Input: part model. Units: mm. Frame: model coordinates. A direction names the side the tool comes from. Give positions to 0.01 mm unless a question says otherwise; leave off trailing zeros. Loops run counter-clockwise (first coordinate to the right, second up) from the corner with the lowest first, then second, coordinate; pieces in that order, holes last. Notation, with made-up numbers: M -6.75,-35 L 30.25,-35 A25 ccw 30.25,0 Z; hole C 51,2.5 d6. An arc over 180 degrees is marked long. Answer as a JSON object with one key per item and string values. Group by question number.
1) Access query for faces 1 (the flat face through (2251.712, 700, 381)), 2 (the flat face through (2251.712, 683, 479)), 3 (the cylindrical face through (2298.4, 703.4, 400)), 4 (the flat face through (2280, 687.227, 517)). Directions: +Z, -Z, +X, -X, +Y, -Y. A direction counts if a zero-diameter tool reaches every point of the face in a straight line with its end or side. Return the directions, or none.
2) Section query D-D on z = 455. Return loops of the section in (x, y).
3) Section query B-B on z = 340.5. Return loops of the section in (x, y).
4) First-contact query: P1, Ø16.5, axis at x = 2271, z = 516.5, coming from the +Y side; P2, Ø10, axis at x = 2292.35, y = 701.47, coming from the +Z side; P3, Ø6, axis at y = 678, z = 319, coming from the +X side; P4, Ø19, axis at x = 2301.5, y = 694, coming from the -Z side. Flat tips, straight axial feed; report the tip coordinate or a pass-through.
5) Section query C-C on z = 275.59. Return loops of the section in (x, y).
6) Section query A-A on x = 2257. Return loops of the section in (y, z), plus the area to 3 significant figures.
7) Draft query along X for faces 5 (the cylindrical face through (2298.4, 703.4, 361.3)), 6 (the flat face through (2260.71, 699.83, 312.56)), 7 (the flat face through (2290.21, 671.3, 451.21)), 8 (the flat face through (2292, 686.862, 328)). Return one class per face: +X half, -X half, draft (parallel to the pull), parting line (faces both ways), or undercut.
8) Ray query, L1, parallel to Z at x = 2275, y = 699; L2, parallel to X at y = 698.5, z = 370.5; L3, parallel to Z at x = 2258.5, y = 714. Return the intervals inside material, ascending.
from build123d import *

# Parameters (mm, degrees)
SKETCH1_R                      = 15
SKETCH1_W                      = 81.28
SKETCH1_H                      = 29.9212
BOSS_EXTRUDE1_DEPTH            = 88.9
CUT_EXTRUDE1_DEPTH             = 894.223960082
CUT_EXTRUDE1_DEPTH_BACK        = 894.223960082
CUT_EXTRUDE2_REACH             = 2404.418
CUT_EXTRUDE2_DIRECTION_2_DEPTH = 2403.418387278
CUT_EXTRUDE3_DEPTH             = 2403.418387278
CUT_EXTRUDE3_DEPTH_BACK        = 31.75
SKETCH6_R                      = 6.35
CUT_EXTRUDE4_DEPTH             = 31.75
SKETCH7_R                      = 6.35
CUT_EXTRUDE5_DEPTH             = 50.8


with BuildPart() as part:
    # Sketch1 → Boss-Extrude1 (new body)
    with BuildSketch(Plane(origin=(0, 718.612000035, 0), x_dir=(1, 0, 0), z_dir=(0, 1, 0))):
        with BuildLine():
            Line((2295.073740346, -527.28515435), (2266.117740346, -527.28515435))
            Line((2266.117740346, -527.28515435), (2241.551712769, -484.433115091))
            Line((2241.551712769, -484.433115091), (2241.551712769, -356.772715091))
            Line((2241.551712769, -356.772715091), (2280.410248463, -267.100940225))
            ThreePointArc((2280.410248463, -267.100940225), (2301.649946984, -254.303850194), (2320.663918503, -270.221111063))
            Line((2320.663918503, -270.221111063), (2343.151712769, -356.772715091))
            Line((2343.151712769, -356.772715091), (2343.151712769, -404.372315091))
            Line((2343.151712769, -404.372315091), (2319.639767922, -484.433115091))
            Line((2319.639767922, -484.433115091), (2295.073740346, -527.28515435))
        make_face()
        with Locations(Location((2299.99999994, -275.59, 0), (0, 0, 270))):
            Circle(SKETCH1_R, mode=Mode.SUBTRACT)
        with Locations((2292.351712769, -380.572515091)):
            Rectangle(SKETCH1_W, SKETCH1_H, mode=Mode.SUBTRACT)
    extrude(amount=-BOSS_EXTRUDE1_DEPTH)

    # Sketch3 → Cut-Extrude1 (cut, two sides: drawn at the far end of the back side and taken through both)
    with BuildSketch(Plane(origin=(2299.99999994, 0, 0), x_dir=(0, 0, -1), z_dir=(1, 0, 0)).offset(-CUT_EXTRUDE1_DEPTH_BACK)):
        Polygon((-254.240000028, 680.512000035), (-414.278315091, 680.512000035), (-489.18515435, 661.827103465), (-527.28515435, 661.827103465), (-527.28515435, 629.712000035), (-254.240000028, 629.712000035), align=None)
        Polygon((-527.28515435, 687.227103465), (-527.28515435, 718.612000035), (-400.308315091, 718.612000035), (-506.96515435, 687.227103465), align=None)
    extrude(amount=CUT_EXTRUDE1_DEPTH + CUT_EXTRUDE1_DEPTH_BACK, mode=Mode.SUBTRACT)

    # Cut-Extrude2: up to this plane
    cut_extrude2_end = Plane(origin=(2241.551712769, 686.673213286, 415.815179194), z_dir=(0, 0.9702698033545601, 0.24202584303810049))
    # Sketch4 → Cut-Extrude2 (cut, up to the surface)
    with BuildSketch(Plane(origin=(0, 718.612000035, 0), x_dir=(1, 0, 0), z_dir=(0, 1, 0)), mode=Mode.PRIVATE) as cut_extrude2_sk1:
        Polygon((2317.374261561, -469.611817535), (2336.533545297, -404.372315091), (2251.711712769, -404.372315091), (2251.711712769, -469.611817535), align=None)
    cut_extrude2_tool1 = split(extrude(cut_extrude2_sk1.sketch, amount=-CUT_EXTRUDE2_REACH, mode=Mode.PRIVATE), bisect_by=cut_extrude2_end, keep=Keep.BOTH, mode=Mode.PRIVATE)
    add(cut_extrude2_tool1.solids().sort_by_distance((2289.536084, 718.612, 435.607712))[0], mode=Mode.SUBTRACT)
    # Sketch4 → Cut-Extrude2 (cut, up to the surface)
    with BuildSketch(Plane(origin=(0, 718.612000035, 0), x_dir=(1, 0, 0), z_dir=(0, 1, 0)), mode=Mode.PRIVATE) as cut_extrude2_sk2:
        Polygon((2313.02160045, -484.433115091), (2315.882386888, -474.691817535), (2251.711712769, -474.691817535), (2251.711712769, -484.433115091), (2264.6287806, -506.96515435), (2300.104532619, -506.96515435), align=None)
    cut_extrude2_tool2 = split(extrude(cut_extrude2_sk2.sketch, amount=-CUT_EXTRUDE2_REACH, mode=Mode.PRIVATE), bisect_by=cut_extrude2_end, keep=Keep.BOTH, mode=Mode.PRIVATE)
    add(cut_extrude2_tool2.solids().sort_by_distance((2282.625495, 718.612, 489.24748))[0], mode=Mode.SUBTRACT)

    # Sketch4 → Cut-Extrude2 direction 2 (cut)
    with BuildSketch(Plane(origin=(0, 718.612000035, 0), x_dir=(1, 0, 0), z_dir=(0, 1, 0))):
        Polygon((2317.374261561, -469.611817535), (2336.533545297, -404.372315091), (2251.711712769, -404.372315091), (2251.711712769, -469.611817535), align=None)
        Polygon((2313.02160045, -484.433115091), (2315.882386888, -474.691817535), (2251.711712769, -474.691817535), (2251.711712769, -484.433115091), (2264.6287806, -506.96515435), (2300.104532619, -506.96515435), align=None)
    extrude(amount=CUT_EXTRUDE2_DIRECTION_2_DEPTH, mode=Mode.SUBTRACT)

    # Sketch5 → Cut-Extrude3 (cut, two sides: drawn at the far end of the back side and taken through both)
    with BuildSketch(Plane(origin=(0, 718.612000035, 0), x_dir=(1, 0, 0), z_dir=(0, 1, 0)).offset(-CUT_EXTRUDE3_DEPTH_BACK)):
        with BuildLine():
            Line((2336.590880718, -356.772715091), (2318.338523091, -286.522569115))
            ThreePointArc((2318.338523091, -286.522569115), (2298.350052896, -296.876149806), (2280.195820512, -283.566025074))
            Line((2280.195820512, -283.566025074), (2248.472295676, -356.772715091))
            Line((2248.472295676, -356.772715091), (2336.590880718, -356.772715091))
        make_face()
    extrude(amount=CUT_EXTRUDE3_DEPTH + CUT_EXTRUDE3_DEPTH_BACK, mode=Mode.SUBTRACT)

    # Sketch6 → Cut-Extrude4 (cut)
    with BuildSketch(Plane.XY.offset(527.28515435)):
        with Locations((2280.595740346, 673.257103465)):
            Circle(SKETCH6_R)
    extrude(amount=-CUT_EXTRUDE4_DEPTH, mode=Mode.SUBTRACT)

    # Sketch7 → Cut-Extrude5 (cut)
    with BuildSketch(Plane.XY.offset(404.372315091)):
        with Locations((2292.351712769, 701.469420385)):
            Circle(SKETCH7_R)
    extrude(amount=-CUT_EXTRUDE5_DEPTH, mode=Mode.SUBTRACT)


solid = part.part
Output:
{
 "1": {"face 1": "+Y, -Y", "face 2": "+Y", "face 3": "none", "face 4": "+Z, +X, -X, +Y"},
 "2": {"outline": "M 2241.55,670.35 L 2328.28,670.35 L 2328.28,702.52 L 2321.67,702.52 L 2321.67,676.9 L 2251.71,676.9 L 2251.71,702.52 L 2241.55,702.52 Z"},
 "3": {"outline": "M 2248.6,680.51 L 2338.92,680.51 L 2338.92,718.61 L 2332.36,718.61 L 2332.36,686.86 L 2255.52,686.86 L 2255.52,718.61 L 2248.6,718.61 Z"},
 "4": {"P1": "stops at y = 687.23", "P2": "stops at z = 474.69", "P3": "stops at x = 2333.76", "P4": "stops at z = 254.24"},
 "5": {"outline": "M 2276.73,680.51 L 2285,680.51 L 2285,718.61 L 2276.73,718.61 Z; M 2315,680.51 L 2322.06,680.51 L 2322.06,718.61 L 2315,718.61 Z"},
 "6": {"outline": "M 661.83,489.19 L 680.51,414.28 L 680.51,395.53 L 718.61,395.53 L 718.61,400.31 L 717.42,404.37 L 689.53,404.37 L 673.25,469.61 L 698.22,469.61 L 696.72,474.69 L 671.99,474.69 L 667.26,493.66 L 691.14,493.66 L 687.23,506.97 L 687.23,511.38 L 661.83,511.38 Z; M 680.51,321.12 L 718.61,321.12 L 718.61,337.09 L 686.86,337.09 L 686.86,356.77 L 718.61,356.77 L 718.61,365.61 L 680.51,365.61 Z", "area": "2,600 mm^2"},
 "7": {"face 5": "undercut", "face 6": "-X half", "face 7": "draft", "face 8": "undercut"},
 "8": {"L1": "z = 279.59 to 295.56, 356.77 to 365.61, 395.53 to 404.37", "L2": "x = 2241.55 to 2251.71, 2332.99 to 2343.15", "L3": "z = 317.66 to 333.63, 356.77 to 365.61, 395.53 to 404.37"}
}
